from build123d import *

# Parameters (mm, degrees)
EXTRUDE_1_DEPTH     = 30
EXTRUDE_START       = 5
EXTRUDE_2_DEPTH     = 5
CUT_EXTRUDE_1_DEPTH = 54.141321022


with BuildPart() as part:
    # Sketch 1 → Extrude 1 (new body)
    with BuildSketch(Plane.XY):
        with BuildLine():
            ThreePointArc((-14, 0), (0, -14), (14, 0))
            Line((14, 0), (8, 0))
            ThreePointArc((8, 0), (0, -8), (-8, 0))
            Line((-8, 0), (-14, 0))
        make_face()
        with BuildLine():
            Line((8, 0), (14, 0))
            ThreePointArc((14, 0), (0, 14), (-14, 0))
            Line((-14, 0), (-8, 0))
            ThreePointArc((-8, 0), (0, 8), (8, 0))
        make_face()
        with BuildLine():
            Line((30, -18), (14, -18))
            Line((14, -18), (14, 0))
            ThreePointArc((14, 0), (0, -14), (-14, 0))
            Line((-14, 0), (-14, -18))
            Line((-14, -18), (-30, -18))
            Line((-30, -18), (-30, -27))
            Line((-30, -27), (30, -27))
            Line((30, -27), (30, -18))
        make_face()
    extrude(amount=-EXTRUDE_1_DEPTH)

    # Sketch 1_3 → Extrude 2 (add)
    with BuildSketch(Plane.XY.offset(EXTRUDE_START)):
        with BuildLine():
            ThreePointArc((-14, 0), (0, -14), (14, 0))
            Line((14, 0), (8, 0))
            ThreePointArc((8, 0), (0, -8), (-8, 0))
            Line((-8, 0), (-14, 0))
        make_face()
        with BuildLine():
            Line((8, 0), (14, 0))
            ThreePointArc((14, 0), (0, 14), (-14, 0))
            Line((-14, 0), (-8, 0))
            ThreePointArc((-8, 0), (0, 8), (8, 0))
        make_face()
    extrude(amount=-EXTRUDE_2_DEPTH)

    # Sketch 2 → Cut-Extrude 1 (cut, through all)
    with BuildSketch(Plane(origin=(0, -18, 0), x_dir=(1, 0, 0), z_dir=(0, 1, 0))):
        with BuildLine():
            Line((30, 10), (22, 10))
            ThreePointArc((22, 10), (17, 15), (22, 20))
            Line((22, 20), (30, 20))
            Line((30, 20), (30, 10))
        make_face()
        with BuildLine():
            Line((-30, 20), (-22, 20))
            ThreePointArc((-22, 20), (-17, 15), (-22, 10))
            Line((-22, 10), (-30, 10))
            Line((-30, 10), (-30, 20))
        make_face()
    extrude(amount=-CUT_EXTRUDE_1_DEPTH, mode=Mode.SUBTRACT)


solid = part.part
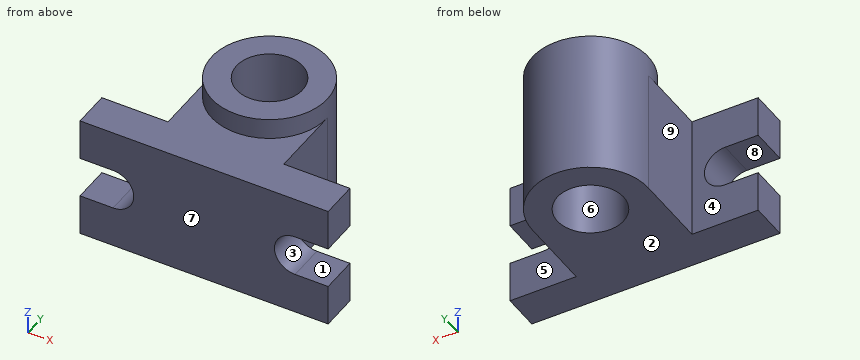
CAD build for the part. Positions are in the model's coordinates, mm. Face numbers are marked on the shaded views. A direction names the side the tool comes from. Give positions to 0.01 mm unless a question says otherwise; leave off trailing zeros. Write each loop counter-clockwise with the first axis right and the second up, starting at its lowest first coordinate (ties: lowest second). Pieces come first, ordered by that corner, then holes. Notation, with made-up numbers: (12, 13.5) -> (51, 13.5) arc R26 cw to (51, 30.5) -> close; hole circle Ø2 at (4.5, -1). An arc over 180 degrees is marked (long way). Return JSON: item names as keys, results as strings.
Item 1: Band-saw the part on A-A (z = -15). List the corners of the cut face in (x, y).
Answer below:
{"outline": "(-17, -27) -> (17, -27) -> (17, -18) -> (14, -18) -> (14, 0) arc R14 ccw to (-14, 0) -> (-14, -18) -> (-17, -18) -> close; hole circle Ø16 at (0, 0)"}
Item 2: Drill centre lines: probe 1 along Y at (x, z) = (-0.5, -2.5); probe 2 along X at (y, z) = (0.5, -22.5); probe 3 along Z at (x, y) = (8.5, -13.5). Where is each one in solid material? Low to high.
Answer below:
{"probe 1": "y = -27 to -7.98, 7.98 to 13.99", "probe 2": "x = -13.99 to -7.98, 7.98 to 13.99", "probe 3": "z = -30 to 0"}
Item 3: Two-plate mould, pull along Z, no slides. Class the marked faces 1, 2, 3 and 4: +Z half, -Z half, draft (parallel to the pull), parting line (faces both ways), or undercut.
Answer below:
{"face 1": "undercut", "face 2": "-Z half", "face 3": "undercut", "face 4": "draft"}
Item 4: Band-saw the part on C-C (y = 3). List the corners of the cut face in (x, z), then the cut area to 3 significant figures.
Answer below:
{"outline": "(-13.67, -30) -> (-7.42, -30) -> (-7.42, 5) -> (-13.67, 5) -> close; (7.42, -30) -> (13.67, -30) -> (13.67, 5) -> (7.42, 5) -> close", "area": "438 mm2"}
Item 5: Drop flat-ended pins along their axis: pin 1 (13 mm diameter, centred on x = 0, y = 0, fed in from -Z); pin 2 (9 mm diameter, centred on x = 25.5, y = -24, fed in from +Z); pin 3 (1 mm diameter, centred on y = 2.5, z = -24.5, fed in from +X); pin 4 (10 mm diameter, centred on x = -21.5, z = -15.5, fed in from +Y). Give the stop position or say it passes through.
Answer below:
{"pin 1": "passes through", "pin 2": "stops at z = 0", "pin 3": "stops at x = 13.86", "pin 4": "stops at y = -18"}
Item 6: Band-saw the part on D-D (z = -3.5). List the corners of the cut face in (x, y), then the cut area to 3 significant figures.
Answer below:
{"outline": "(-30, -27) -> (30, -27) -> (30, -18) -> (14, -18) -> (14, 0) arc R14 ccw to (-14, 0) -> (-14, -18) -> (-30, -18) -> close; hole circle Ø16 at (0, 0)", "area": "1,150 mm2"}
Item 7: Band-saw the part on B-B (x = 0). List the corners of the cut face in (y, z).
Answer below:
{"outline": "(-27, -30) -> (-8, -30) -> (-8, 5) -> (-14, 5) -> (-14, 0) -> (-27, 0) -> close; (8, -30) -> (14, -30) -> (14, 5) -> (8, 5) -> close"}
Item 8: Tool access for the marked faces 5, 6, 7, 8 and 9: list every direction of +Z, -Z, +X, -X, +Y, -Y with a clear straight run to the whole face (end or side of a thin tool).
Answer below:
{"face 5": "+Z, -Z, +X, +Y", "face 6": "+Z, -Z", "face 7": "+Z, -Z, +X, -X, -Y", "face 8": "-X, +Y, -Y", "face 9": "+Z, -Z, -X, +Y"}
